The listing builds one solid part. Answer for the finished solid, in the listing's coordinates (mm). Round coordinates to 2 decimals unless told otherwise and drop trailing zeros. Loops run counter-clockwise (first coordinate to the right, second up) from the corner with the lowest first, then second, coordinate; pieces in that order, holes last. Notation, with made-up numbers: (-21.75, 63) -> (9.25, 63) arc R24 cw to (9.25, 75) -> close; hole circle Ø8 at (31.25, -24). An arc over 180 degrees is marked (long way). Write each question's results on one line, items separated by ' | '. Start each with the question number.
(1) The part is cut by section C-C (z = 37). Determine the outline of the cut face in (x, y).
(2) The part is cut by section B-B (x = -33). Determine the outline of the cut face in (y, z).
(3) Straight lines are drawn through the part: probe 1 along Z at (x, y) = (0, 19); probe 2 along Y at (x, z) = (2, -38); probe 3 along Z at (x, y) = (0, -1). For each, find the intervals that lie inside material, in ascending order.
(4) The part is cut by section D-D (y = 22). Determine the outline of the cut face in (x, z).
(5) The part is cut by section A-A (z = 0). Determine the outline of the cut face in (x, y), plus the area to 3 significant figures.
(6) Flat-ended cylindrical pins translate along their axes: pin 1 (3 mm diameter, centred on x = 14.5, y = 6.5, fed in from +Z); pin 2 (1.5 mm diameter, centred on y = 21, z = -13.5, fed in from -X); pin 3 (1 mm diameter, centred on y = 24.5, z = 13.5, fed in from -X). Find the tip coordinate at first contact, or state that the pin passes through.
Autodesk Inventor part; units mm, degrees
ref_plane "YZ Plane" through (0, 0, 0) normal (1, 0, 0) x (0, 1, 0)
ref_plane "XZ Plane" through (0, 0, 0) normal (0, 1, 0) x (-1, 0, 0)
ref_plane "XY Plane" through (0, 0, 0) normal (0, 0, 1) x (1, 0, 0)
sketch "Sketch1" plane through (0, 0, 0) normal (0, 0, 1) x (1, 0, 0)
  line L0 (-40, 0) -> (-40, 32)
  line L1 (-42, 34) -> (-42, -2)
  line L2 (-40, 0) -> (0, 0)
  line L3 (0, 0) -> (0, -2)
  line L4 (0, -2) -> (-42, -2)
  line L5 (0, -10.8) -> (0, 50.8)
  line L6 (-42, 34) -> (0, 34)
  line L7 (-40, 32) -> (0, 32)
  line L8 (0, 32) -> (0, 34)
  dimension "d5" = 2
  dimension "radius" = 40
  dimension "d7" = 2
  dimension "d37" = 2
  dimension "SampleVolumeInnerHeight" = 32
revolve "Revolution1" add sketch "Sketch1" angle 360 about axis through (0, -10, 0) along (0, 1, 0) contours L2 L3 L4 L1 L6 L5 L7 L0
sketch "Sketch3" plane through (0, -2, 0) normal (0, -1, 0) x (1, 0, 0)
  line L0 (-12.4915, 0) -> (12.0084, 0)
  point P0 (0, 0)
  dimension "DistanceBetweenHolesSweep" = 24.5
hole "Hole2" at (0, -2, 0) direction (0, 1, 0) diameter 5.08 depth 2
hole "Hole3" at (-12.4915, -2, 0) at (12.0084, -2, 0) direction (0, 1, 0) diameter 5 depth 2
equation "\"d5\" = thickness"
equation "\"radius\" = 0.5 * SaltDiameter"
equation "\"d7\" = thickness"
equation "\"d37\" = crucible_thickness"
equation "\"SampleVolumeInnerHeight\" = 4 * SaltThickness"
equation "\"d22\" = fixation_holes_diameter"
equation "\"d30\" = PenetrationOuterDiameter"
equation "\"thickness\" = crucible_thickness"
properties part number "UpstreamVolume" material "Nickel-Copper Alloy 400"
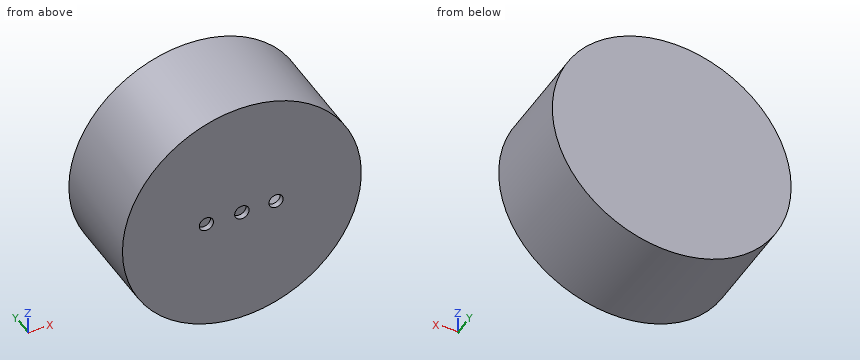
Checked values:
1) outline: (-19.87, -2) -> (19.87, -2) -> (19.87, 34) -> (-19.87, 34) -> close; hole (-15.2, 0) -> (15.2, 0) -> (15.2, 32) -> (-15.2, 32) -> close
2) outline: (-2, -25.98) -> (34, -25.98) -> (34, 25.98) -> (-2, 25.98) -> close; hole (0, -22.61) -> (32, -22.61) -> (32, 22.61) -> (0, 22.61) -> close
3) probe 1: z = -42 to -40, 40 to 42 | probe 2: y = -2 to 0, 32 to 34 | probe 3: z = -42 to -2.54, 2.54 to 42
4) outline: circle Ø84 at (0, 0); hole circle Ø80 at (0, 0)
5) outline: (-42, -2) -> (-14.99, -2) -> (-14.99, 0) -> (-40, 0) -> (-40, 32) -> (40, 32) -> (40, 0) -> (14.51, 0) -> (14.51, -2) -> (42, -2) -> (42, 34) -> (-42, 34) -> close; (-9.99, -2) -> (-2.54, -2) -> (-2.54, 0) -> (-9.99, 0) -> close; (2.54, -2) -> (9.51, -2) -> (9.51, 0) -> (2.54, 0) -> close | area: 434 mm2
6) pin 1: stops at z = 39.94 | pin 2: stops at x = -40.02 | pin 3: stops at x = -39.94
